Check sheet for the drawn part. Datum: minimum x, y, z corner. Units: mm. Coordinates: 2 decimals unless noted, no trailing zeros. Order: outer loops, then holes, each group sorted by start corner. A loop starts at its lowest first (then second) coordinate and runs counter-clockwise, first axis right, second up. Notation, with made-up numbers: (84.5, 47.5) - (90.5, 47.5) arc R27 cw to (90.5, 82.5) - close; hole circle Ø6 at (-35.75, 35). An arc over 180 degrees is marked (long way). Return JSON: item names as keys, results as strings. Group by question number.
Item 1: Section check C-C on y = 30.5. Enter the section's corners in (x, z), then the cut area to 3 significant figures.
Item 2: Scan lines: probe 1 along Y at (x, z) = (3.75, 20) (1 decimal); probe 2 along Y at (x, z) = (2.5, 11); probe 3 along Y at (x, z) = (5, 12.5). Record each from-to range of solid material in increasing order.
Item 3: Section check A-A on y = 19.5. Enter the section's corners in (x, z), then the cut area to 3 significant figures.
Item 4: Draft check along Y on the marked faces 1, 2 and 3. Enter one of: pulls with the +Y half, pulls with the -Y half, needs draft (parallel to the pull), parting line crosses it, or undercut.
Item 5: Section check D-D on x = 6. Enter the section's corners in (y, z).
Item 6: Section check B-B on x = 2. Enter the section's corners in (y, z).
Item 7: Gauge pin test, flat ends, axial feed: pin 1 (19.5 mm diameter, centred on y = 18.5, z = 17, fed in from -X); pin 2 (3 mm diameter, centred on x = 2, z = 12.5, fed in from -Y); pin 3 (1.5 mm diameter, centred on y = 28.5, z = 5, fed in from -X); pin 4 (1.5 mm diameter, centred on x = 2.5, z = 13.5, fed in from -Y). Record the tip position at first contact, or that the pin passes through.
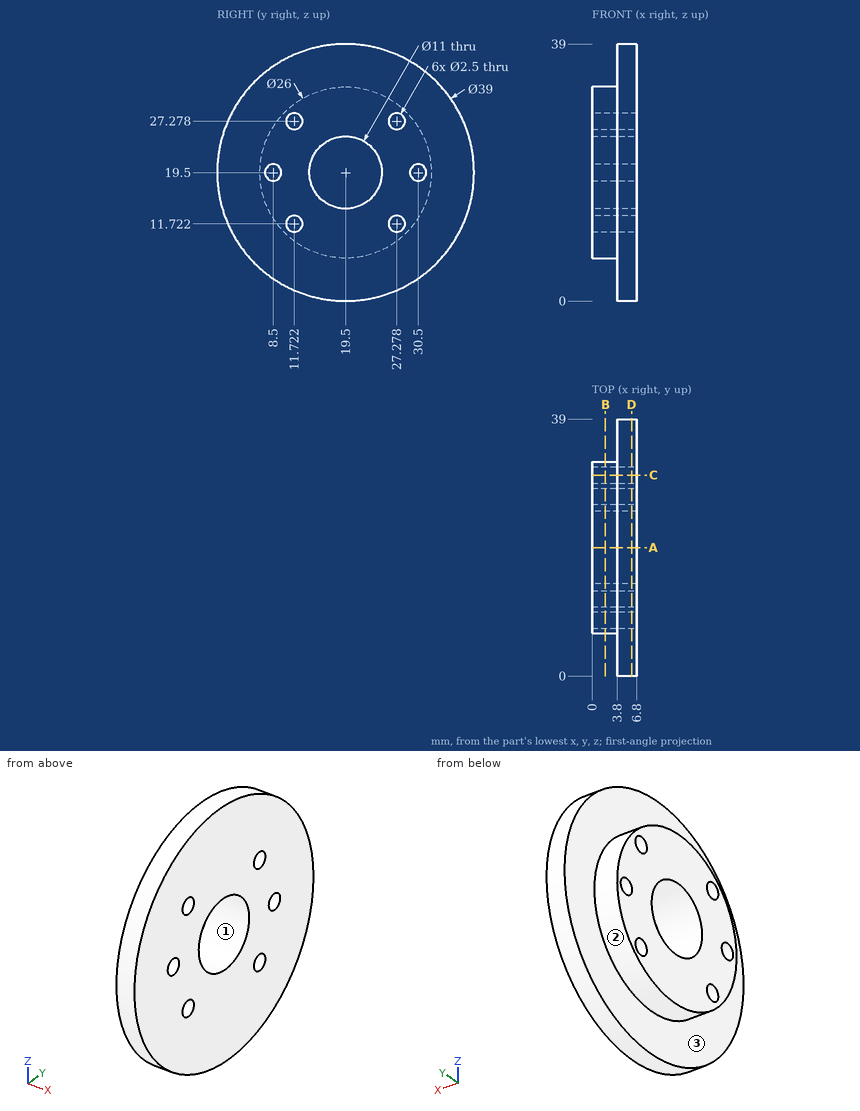
Computed:
{
 "1": {"outline": "(0, 12.57) - (3.8, 12.57) - (3.8, 3.4) - (6.8, 3.4) - (6.8, 18.25) - (0, 18.25) - close; (0, 20.75) - (6.8, 20.75) - (6.8, 35.6) - (3.8, 35.6) - (3.8, 26.43) - (0, 26.43) - close", "area": "132 mm²"},
 "2": {"probe 1": "y = 6.5 to 7.4, 9.6 to 14, 25 to 29.4, 31.6 to 32.5", "probe 2": "y = 9.66 to 10.7, 12.74 to 26.26, 28.3 to 29.34", "probe 3": "y = 1.3 to 10.74, 12.7 to 26.3, 28.26 to 37.7"},
 "3": {"outline": "(0, 6.5) - (3.8, 6.5) - (3.8, 0) - (6.8, 0) - (6.8, 14) - (0, 14) - close; (0, 25) - (6.8, 25) - (6.8, 39) - (3.8, 39) - (3.8, 32.5) - (0, 32.5) - close", "area": "141 mm²"},
 "4": {"face 1": "undercut", "face 2": "parting line crosses it", "face 3": "needs draft"},
 "5": {"outline": "circle Ø39 at (19.5, 19.5); hole circle Ø2.5 at (8.5, 19.5); hole circle Ø2.5 at (11.72, 11.72); hole circle Ø2.5 at (11.72, 27.28); hole circle Ø11 at (19.5, 19.5); hole circle Ø2.5 at (27.28, 11.72); hole circle Ø2.5 at (27.28, 27.28); hole circle Ø2.5 at (30.5, 19.5)"},
 "6": {"outline": "circle Ø26 at (19.5, 19.5); hole circle Ø2.5 at (8.5, 19.5); hole circle Ø2.5 at (11.72, 11.72); hole circle Ø2.5 at (11.72, 27.28); hole circle Ø11 at (19.5, 19.5); hole circle Ø2.5 at (27.28, 11.72); hole circle Ø2.5 at (27.28, 27.28); hole circle Ø2.5 at (30.5, 19.5)"},
 "7": {"pin 1": "stops at x = 0", "pin 2": "stops at y = 7.72", "pin 3": "stops at x = 3.8", "pin 4": "stops at y = 7.61"}
}
